Geometry: final body of the model. Coordinates: model frame, mm. A direction names the side the tool comes from. Round coordinates to 2 decimals unless told otherwise and drop trailing zeros. Loops run counter-clockwise (first coordinate to the right, second up) from the corner with the lowest first, then second, coordinate; pieces in that order, holes last. Notation, with made-up numbers: (61, 12) - (78, 12) arc R19 cw to (78, 35) - close; hole circle Ø7 at (-14, 78.5). An arc over 180 degrees is marked (long way). Answer as a JSON object with one key per item and string values. Group by question number.
Item 1: Line query: line 1 (Z direction, x = -1.5, y = 3.5); line 2 (X direction, y = 12, z = -4); line 3 (Y direction, x = 17.5, z = -7). Output: solid intervals per line, ascending.
Item 2: First-contact query: pin 1 (5 mm diameter, centred on x = -19, y = 8, fed in from +Z); pin 2 (3 mm diameter, centred on x = -19, y = 8, fed in from -Z); pin 3 (2 mm diameter, centred on x = 8.5, y = 4.5, fed in from -Z). Flat tips, straight axial feed; report the tip coordinate or a pass-through.
Item 3: Section A-A (x = -18.5). Return the cut outline in (y, z), plus the area to 3 significant figures.
Item 4: Reachability of faces 5 (the face through (-20, 11.43, 0)), 6 (the face through (-1, 9, -32.088)), 7 (the face through (-1, 9, 32.682)), 8 (the face through (19, 6, -30.31)) from +Z, -Z, +X, -X, +Y, -Y: full face, straight path, thin tool, end or side. Return the list, or none.
Item 5: Section B-B (y = 10.25). Return the cut outline in (x, z), plus the area to 3 significant figures.
Item 6: Draft query along Z for faces 1 (the face through (22.411, 0.501, -34.877)), 2 (the face through (13.776, 13, 0)), 3 (the face through (-20, 6, -30.31)), 4 (the face through (-20, 6, 30.904)). Return one class per face: released by +Z, released by -Z, zero draft, split by the parting line, or undercut.
Item 7: Section C-C (z = -17). Return the cut outline in (x, y).
```python
from build123d import *

# Parameters (mm, degrees)
SKETCH1_W           = 28.702
SKETCH1_H           = 64.77
BOSS_EXTRUDE1_DEPTH = 16.51
SKETCH1_6_W         = 10.414
SKETCH1_6_H         = 61.214
BOSS_EXTRUDE2_DEPTH = 11.43
SKETCH1_7_R         = 1.651
BOSS_EXTRUDE3_DEPTH = 1.016


with BuildPart() as part:
    # Sketch1 → Boss-Extrude1 (new body)
    with BuildSketch(Plane(origin=(0, 0, 0), x_dir=(1, 0, 0), z_dir=(0, 1, 0))):
        with Locations((-0.574727978, -0.297335239)):
            Rectangle(SKETCH1_W, SKETCH1_H)
    extrude(amount=BOSS_EXTRUDE1_DEPTH)

    # Sketch1_6 → Boss-Extrude2 (add)
    with BuildSketch(Plane(origin=(0, 0, 0), x_dir=(1, 0, 0), z_dir=(0, 1, 0))):
        with Locations((-20.132727978, -0.297335239)):
            Rectangle(SKETCH1_6_W, SKETCH1_6_H)
        with Locations((18.983272022, -0.297335239)):
            Rectangle(SKETCH1_6_W, SKETCH1_6_H)
    extrude(amount=BOSS_EXTRUDE2_DEPTH)

    # Sketch1_7 → Boss-Extrude3 (add)
    with BuildSketch(Plane(origin=(0, 0, 0), x_dir=(1, 0, 0), z_dir=(0, 1, 0))):
        Polygon((-25.339727978, 36.151664761), (-25.339727978, 30.309664761), (-14.925727978, 30.309664761), (-14.925727978, 32.087664761), (13.776272022, 32.087664761), (13.776272022, 30.309664761), (24.190272022, 30.309664761), (24.190272022, 36.151664761), align=None)
        with Locations((-22.672727978, 33.484664761)):
            Circle(SKETCH1_7_R, mode=Mode.SUBTRACT)
        with Locations((21.523272022, 33.484664761)):
            Circle(SKETCH1_7_R, mode=Mode.SUBTRACT)
        Polygon((-14.925727978, -30.904335239), (-25.339727978, -30.904335239), (-25.339727978, -36.746335239), (24.190272022, -36.746335239), (24.190272022, -30.904335239), (13.776272022, -30.904335239), (13.776272022, -32.682335239), (-14.925727978, -32.682335239), align=None)
        with Locations((-22.672727978, -34.079335239)):
            Circle(SKETCH1_7_R, mode=Mode.SUBTRACT)
        with Locations((21.523272022, -34.079335239)):
            Circle(SKETCH1_7_R, mode=Mode.SUBTRACT)
    extrude(amount=BOSS_EXTRUDE3_DEPTH)


solid = part.part
```
Values:
{
 "1": {"line 1": "z = -32.09 to 32.68", "line 2": "x = -14.93 to 13.78", "line 3": "y = 0 to 11.43"},
 "2": {"pin 1": "stops at z = 30.9", "pin 2": "stops at z = -30.31", "pin 3": "stops at z = -32.09"},
 "3": {"outline": "(0, -36.15) - (1.02, -36.15) - (1.02, -30.31) - (11.43, -30.31) - (11.43, 30.9) - (1.02, 30.9) - (1.02, 36.75) - (0, 36.75) - close", "area": "712 mm^2"},
 "4": {"face 5": "+Z, -Z, -X, +Y", "face 6": "-Z, +X, -X, +Y", "face 7": "+Z, +X, -X, +Y", "face 8": "-Z, +X, +Y"},
 "5": {"outline": "(-25.34, -30.31) - (-14.93, -30.31) - (-14.93, -32.09) - (13.78, -32.09) - (13.78, -30.31) - (24.19, -30.31) - (24.19, 30.9) - (13.78, 30.9) - (13.78, 32.68) - (-14.93, 32.68) - (-14.93, 30.9) - (-25.34, 30.9) - close", "area": "3,130 mm^2"},
 "6": {"face 1": "undercut", "face 2": "zero draft", "face 3": "released by -Z", "face 4": "released by +Z"},
 "7": {"outline": "(-25.34, 0) - (24.19, 0) - (24.19, 11.43) - (13.78, 11.43) - (13.78, 16.51) - (-14.93, 16.51) - (-14.93, 11.43) - (-25.34, 11.43) - close"}
}
